Design review of the part built by this model. Coordinates are the model's own, in mm. Face numbers are marked on the shaded views. A direction names the side the tool comes from. Coordinates: 2 decimals unless noted, no trailing zeros. Loops run counter-clockwise (first coordinate to the right, second up) from the corner with the lowest first, then second, coordinate; pieces in that order, holes last.
from build123d import *

# Parameters (mm, degrees)
PAD_DEPTH    = 1.6
PAD001_DEPTH = 1
FILLET_R     = 1
FILLET002_R  = 0.59
FILLET003_R  = 0.59


with BuildPart() as part:
    # Sketch → Pad (new body)
    with BuildSketch(Plane.XY):
        Polygon((0, 10), (-1.5, 10), (-1.5, -1.2), (10, -1.2), (10, 0), (0, 0), align=None)
    extrude(amount=PAD_DEPTH)

    # Sketch001 → Pad001 (join)
    with BuildSketch(Plane.XY):
        Polygon((-1.5, 10), (-1.5, -1.2), (10, -1.2), (10, 0), (0, 10), align=None)
    extrude(amount=-PAD001_DEPTH)

    # Fillet
    fillet_edges = [part.edges().sort_by_distance(p)[0] for p in [
        (-1.5, -1.2, 0.3),
    ]]
    fillet(fillet_edges, radius=FILLET_R)

    # Fillet002
    fillet002_edges = [part.edges().sort_by_distance(p)[0] for p in [
        (0, 10, 0.8),
        (10, -1.2, 0.3),
        (10, 0, 0.8),
        (-1.5, 10, 0.3),
    ]]
    fillet(fillet002_edges, radius=FILLET002_R)

    # Fillet003
    fillet003_edges = [part.edges().sort_by_distance(p)[0] for p in [
        (10, 0, -0.5),
        (0, 10, -0.5),
    ]]
    fillet(fillet003_edges, radius=FILLET003_R)


solid = part.part
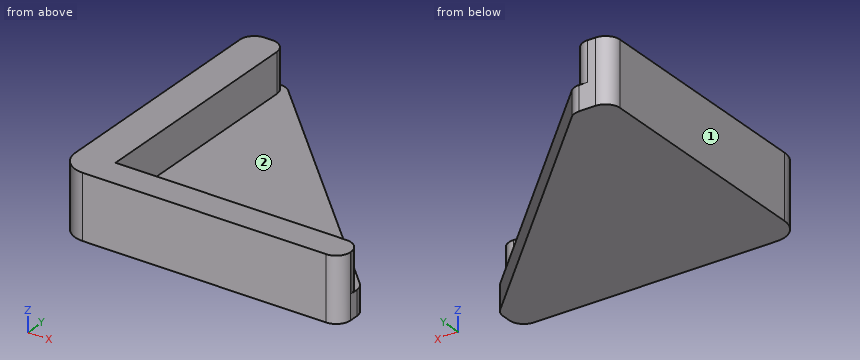
Q1. Take a section at B-B, the plane y = 3.5. Write out the cut boundary in (x, z).
Q2. Clearance check with a flat-ended pin moving along its axis: pin 1 Ø3 at (x, y) = (6.5, 6.5) entering from +Z. State where the tip first meets the part, or that it passes through.
Q3. Machinability: for the marked faces 1 and 2, which of the approach directions +Z, -Z, +X, -X, +Y, -Y give a long, thin tool a straight path to every point of the face, cutting with its end or side? Answer none if there is none.
Q4. Take a section at C-C, the plane x = 7.5. Write out the cut boundary in (y, z).
Q5. For line 1 (Z direction, x = 6.25, y = 3); line 2 (Y direction, x = 7.5, z = 0.4); line 3 (X direction, y = 1.5, z = 0.45), list the stretches that pass through material, from the lowest coordinate up.
Entries:
1. outline: (-1.5, -1) - (6.5, -1) - (6.5, 0) - (0, 0) - (0, 1.6) - (-1.5, 1.6) - close
2. pin 1: passes through
3. face 1: +Z, -Z, -X, +Y, -Y
3. face 2: +Z, +X, +Y
4. outline: (-1.2, -1) - (2.5, -1) - (2.5, 0) - (0, 0) - (0, 1.6) - (-1.2, 1.6) - close
5. line 1: z = -1 to 0
5. line 2: y = -1.2 to 0
5. line 3: x = -1.5 to 0
